```python
from build123d import *

# Parameters (mm, degrees)
BOSS_EXTRUDE1_DEPTH                                 = 17.78
CBORE_FOR_00_BINDING_HEAD_MACHINE_SCREW_D           = 13.4874
CBORE_FOR_00_BINDING_HEAD_MACHINE_SCREW_CBORE_D     = 23.876
CBORE_FOR_00_BINDING_HEAD_MACHINE_SCREW_CBORE_DEPTH = 1.016
SKETCH4_R                                           = 12.7
BOSS_EXTRUDE2_DEPTH                                 = 19.05
F_1_8_0_125_DIAMETER_HOLE1_REACH                    = 115.628
F_1_8_0_125_DIAMETER_HOLE1_BORE_R                   = 1.5875
FILLET1_R                                           = 2.54


with BuildPart() as part:
    # Sketch1 → Boss-Extrude1 (new body)
    with BuildSketch(Plane(origin=(0, 0, 0), x_dir=(1, 0, 0), z_dir=(0, 1, 0))):
        with BuildLine():
            Line((63.246, 22.032212417), (10.16, 36.720354029))
            ThreePointArc((10.16, 36.720354029), (0, 38.1), (-10.16, 36.720354029))
            Line((-10.16, 36.720354029), (-63.246, 22.032212417))
            ThreePointArc((-63.246, 22.032212417), (-80.01, 0), (-63.246, -22.032212417))
            Line((-63.246, -22.032212417), (-10.16, -36.720354029))
            ThreePointArc((-10.16, -36.720354029), (0, -38.1), (10.16, -36.720354029))
            Line((10.16, -36.720354029), (63.246, -22.032212417))
            ThreePointArc((63.246, -22.032212417), (80.01, 0), (63.246, 22.032212417))
        make_face()
    extrude(amount=BOSS_EXTRUDE1_DEPTH)

    # CBORE for #00 Binding Head Machine Screw1 (through all)
    with Locations(Plane(origin=(0, 17.78, 0), x_dir=(1, 0, 0), z_dir=(0, 1, 0))):
        with Locations((-57.15, 0), (57.15, 0)):
            CounterBoreHole(CBORE_FOR_00_BINDING_HEAD_MACHINE_SCREW_D / 2, CBORE_FOR_00_BINDING_HEAD_MACHINE_SCREW_CBORE_D / 2, CBORE_FOR_00_BINDING_HEAD_MACHINE_SCREW_CBORE_DEPTH)

    # Sketch4 → Boss-Extrude2 (add, symmetric)
    with BuildSketch(Plane(origin=(0, 0, 0), x_dir=(0, -1, 0), z_dir=(0.7071067811865464, 0, 0.7071067811865488))):
        with BuildLine():
            Line((-45.72, 25.4), (-15.24, 25.4))
            Line((-15.24, 25.4), (-15.24, -25.4))
            Line((-15.24, -25.4), (-45.72, -25.4))
            ThreePointArc((-45.72, -25.4), (-71.12, 0), (-45.72, 25.4))
        make_face()
        with Locations(Location((-45.72, 0, 0), (0, 0, 90))):
            Circle(SKETCH4_R, mode=Mode.SUBTRACT)
    extrude(amount=BOSS_EXTRUDE2_DEPTH, both=True)

    # 1/8 (0.125) Diameter Hole1 bore (on position points) → 1/8 (0.125) Diameter Hole1 (cut, up to next)
    with BuildSketch(Plane.ZX.offset(71.12), mode=Mode.PRIVATE) as f_1_8_0_125_diameter_hole1_sk1:
        Circle(F_1_8_0_125_DIAMETER_HOLE1_BORE_R)
    f_1_8_0_125_diameter_hole1_tool1 = extrude(f_1_8_0_125_diameter_hole1_sk1.sketch, amount=-F_1_8_0_125_DIAMETER_HOLE1_REACH, mode=Mode.PRIVATE) & part.part
    add(f_1_8_0_125_diameter_hole1_tool1.solids().sort_by_distance((0, 71.12, 0))[0], mode=Mode.SUBTRACT)

    # Fillet1
    fillet1_edges = [part.edges().sort_by_distance(p)[0] for p in [
        (0, 17.78, -38.1),
        (-36.703, 17.78, -29.376283223),
        (-80.01, 17.78, 0),
        (-36.703, 17.78, 29.376283223),
        (0, 17.78, 38.1),
        (36.703, 17.78, 29.376283223),
        (80.01, 17.78, 0),
        (17.960512242, 17.78, -17.960512242),
        (-13.470384182, 17.78, -13.470384182),
        (13.470384182, 17.78, 13.470384182),
        (-17.960512242, 17.78, 17.960512242),
        (-4.490128061, 31.75, 31.430896424),
        (31.430896424, 31.75, -4.490128061),
        (13.470384182, 71.12, 13.470384182),
        (-13.470384182, 71.12, -13.470384182),
        (-31.430896424, 31.75, 4.490128061),
        (4.490128061, 31.75, -31.430896424),
        (36.703, 17.78, -29.376283223),
    ]]
    fillet(fillet1_edges, radius=FILLET1_R)


solid = part.part
```
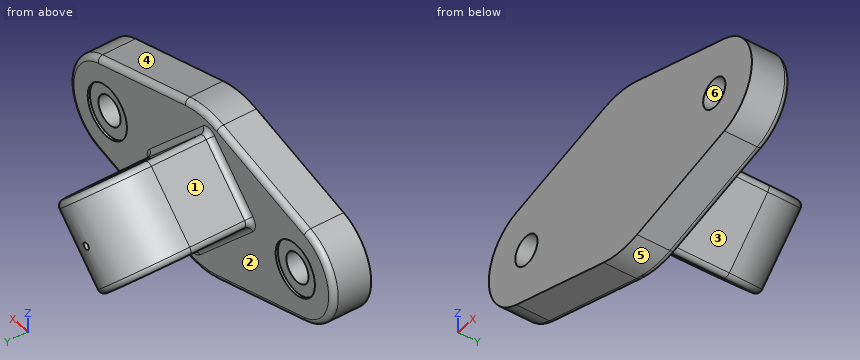
The model under review builds one solid part; all positions refer to its coordinate system, in mm. Face numbers are marked on the shaded views. A direction names the side the tool comes from. Round coordinates to 2 decimals unless told otherwise and drop trailing zeros. Write each loop counter-clockwise with the first axis right and the second up, starting at its lowest first coordinate (ties: lowest second). Pieces come first, ordered by that corner, then holes. Notation, with made-up numbers: (33.5, 17.5) - (61.5, 17.5) arc R20 cw to (61.5, 43.5) - close; hole circle Ø4 at (37, -33). An arc over 180 degrees is marked (long way). Use one line per item in the form item = value.
Q1. Draft analysis for pull direction X (two halves, no side actions). For the marked faces 4, 5 and 6, state which applies: +X half, -X half, draft (parallel to the pull), parting line (faces both ways), or undercut.
Answer key:
face_4 = +X half
face_5 = parting line
face_6 = undercut
Q2. Tool access review of the marked faces 1, 2 and 3: name each direction out of +Z, -Z, +X, -X, +Y, -Y from which nothing blocks a thin tool from reaching the whole face with its end or side.
Answer key:
face_1 = +Z, -X, +Y
face_2 = +Y
face_3 = -Z, +X, +Y
Q3. Consider section A-A (y = 10). State the section outline as (x, z) points, and give its area (3 significant figures).
Answer key:
outline = (-63.25, -22.03) - (-10.16, -36.72) arc R38.1 ccw to (10.16, -36.72) - (63.25, -22.03) arc R22.86 ccw to (63.25, 22.03) - (10.16, 36.72) arc R38.1 ccw to (-10.16, 36.72) - (-63.25, 22.03) arc R22.86 ccw to start; hole circle Ø13.49 at (-57.15, 0); hole circle Ø13.49 at (57.15, 0)
area = 8,570 mm2
Q4. Consider section B-B (y = 43). State the section outline as (x, z) points.
Answer key:
outline = (-29.63, 2.69) - (-22.24, -4.7) - (4.7, 22.24) - (-2.69, 29.63) arc R2.54 ccw to (-6.29, 29.63) - (-29.63, 6.29) arc R2.54 ccw to start; (-4.7, -22.24) - (2.69, -29.63) arc R2.54 ccw to (6.29, -29.63) - (29.63, -6.29) arc R2.54 ccw to (29.63, -2.69) - (22.24, 4.7) - close
Q5. Insertion check: pin 1 Ø4 at (y, z) = (14, 18.5) entering from +X; pin 2 Ø1.5 at (y, z) = (30.5, -25.5) entering from -X; pin 3 Ø21.5 at (x, z) = (16, 0) entering from +Y. Each pin has a flat end and moves straight along its axis. Give the tip position at first contact, or say it passes through.
Answer key:
pin_1 = 72.97
pin_2 = -2.19
pin_3 = 71.11
Q6. Consider section C-C (y = 29). State the section outline as (x, z) points.
Answer key:
outline = (-29.63, 2.69) - (2.69, -29.63) arc R2.54 ccw to (6.29, -29.63) - (29.63, -6.29) arc R2.54 ccw to (29.63, -2.69) - (-2.69, 29.63) arc R2.54 ccw to (-6.29, 29.63) - (-29.63, 6.29) arc R2.54 ccw to start
Q7. For line 1 (X direction, y = 67, z = 0); line 2 (Y direction, x = 27, z = 15); line 3 (X direction, y = 55, z = -28.5), list the stretches that pass through material, from the lowest coordinate up. Write a range as [from, to].
Answer key:
line_1 = [-19.61, -1.59], [1.59, 19.61]
line_2 = [0, 17.78]
line_3 = [1.59, 4.93]
